Source: CAD feature listing. Evaluate the final solid. Frame: model axes, mm. Face numbers are marked on the shaded views. A direction names the side the tool comes from. Coordinates: 2 decimals unless noted, no trailing zeros. Order: outer loops, then holes, each group sorted by start corner. A loop starts at its lowest first (then second) coordinate and runs counter-clockwise, first axis right, second up. Notation, with made-up numbers: (18, -23) - (53, -23) arc R30 cw to (53, 9) - close; hole circle Ø8 at (19.25, 39.25). An arc over 180 degrees is marked (long way). One line per question, with ' | ' between items. Start each with the question number.
(1) Section B-B (z = 4.5). Count the separate pieces of the cut face and the enclosed holes in it, then the cut area to 3 significant figures.
(2) Section A-A (y = 0). Return the cut outline in (x, z), then the cut area to 3 significant figures.
(3) Contact query for flat-ended pins moving along their axis: P1, Ø2, axis at x = 9, y = 8, coming from the -Z side; P2, Ø5, axis at y = -14.5, z = 2, coming from the -X side; P3, Ø6.5, axis at y = 1, z = -0.5, coming from the +X side. Output: stop coordinate, or through.
(4) Access query for the marked faces 5 and 6. Directions: +Z, -Z, +X, -X, +Y, -Y. A direction counts if a zero-diameter tool reaches every point of the face in a straight line with its end or side. Return the directions, or none.
(5) Draft query along Y for the marked faces 1, 2, 3 and 4. Return one class per face: +Y half, -Y half, draft (parallel to the pull), parting line (faces both ways), or undercut.
(6) Line query: line 1 along Z through (x, y) = (-5.55, 0); line 2 along Y through (x, z) = (7, 5.25); line 3 along Y through (x, z) = (13.5, -1.25). Output: solid intervals per line, ascending.
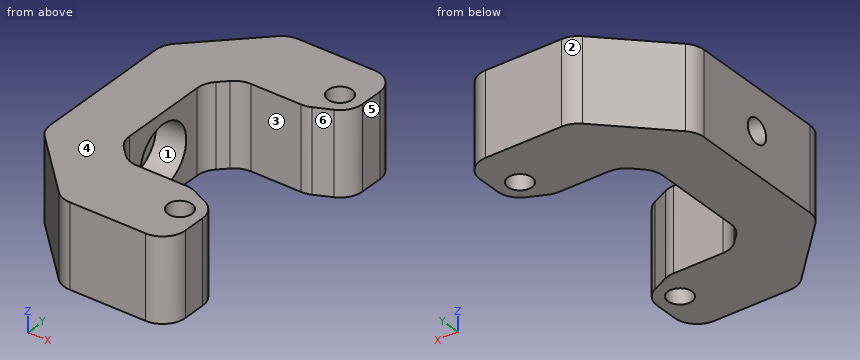
from build123d import *

# Parameters (mm, degrees)
SKETCH_R             = 1.6
PAD_DEPTH            = 5.5
SKETCH001_R          = 1.6
POCKET_DEPTH         = 8.001
POCKET001_DEPTH      = 5.501
POCKET001_DEPTH_BACK = 5.501
SKETCH003_W          = 10
SKETCH003_H          = 45
POCKET002_DEPTH      = 5.501
POCKET002_DEPTH_BACK = 5.501
SKETCH004_R          = 4
POCKET003_DEPTH      = 4
FILLET_R             = 3


with BuildPart() as part:
    # Sketch → Pad (new body, symmetric)
    with BuildSketch(Plane.XY):
        Polygon((1.514719, 20), (18.828427, 20), (18.828427, 10), (6.828427, 10), (2.828427, 10), (0, 7.171573), (0, -7.171573), (2.828427, -10), (6.828427, -10), (18.828427, -10), (18.828427, -20), (1.514719, -20), (-8, -10.485281), (-8, 10.485281), align=None)
        with Locations((12.828427, 14)):
            Circle(SKETCH_R, mode=Mode.SUBTRACT)
        with Locations((12.828427, -14)):
            Circle(SKETCH_R, mode=Mode.SUBTRACT)
    extrude(amount=PAD_DEPTH, both=True)

    # Sketch001 → Pocket (cut, through all)
    with BuildSketch(Plane.YZ):
        Circle(SKETCH001_R)
    extrude(amount=-POCKET_DEPTH, mode=Mode.SUBTRACT)

    # Sketch002 → Pocket001 (cut, two sides)
    with BuildSketch(Plane.XY) as pocket001_sk:
        Polygon((18.828427, 13.487712), (11.349004, 10), (18.828427, 10), align=None)
        Polygon((11.349004, -10), (18.828427, -13.487712), (18.828427, -10), align=None)
    extrude(amount=-POCKET001_DEPTH, mode=Mode.SUBTRACT)
    extrude(pocket001_sk.sketch, amount=POCKET001_DEPTH_BACK, mode=Mode.SUBTRACT)

    # Sketch003 → Pocket002 (cut, two sides)
    with BuildSketch(Plane.XY) as pocket002_sk:
        with Locations((20.828427, 0)):
            Rectangle(SKETCH003_W, SKETCH003_H)
    extrude(amount=-POCKET002_DEPTH, mode=Mode.SUBTRACT)
    extrude(pocket002_sk.sketch, amount=POCKET002_DEPTH_BACK, mode=Mode.SUBTRACT)

    # Sketch004 → Pocket003 (cut)
    with BuildSketch(Plane.YZ):
        Circle(SKETCH004_R)
    extrude(amount=-POCKET003_DEPTH, mode=Mode.SUBTRACT)

    # Fillet
    fillet_edges = [part.edges().sort_by_distance(p)[0] for p in [
        (15.828427, -20, 0),
        (15.828427, -12.088789, 0),
        (11.349004, -10, 0),
        (2.828427, -10, 0),
        (0, -7.171573, 0),
        (0, 7.171573, 0),
        (2.828427, 10, 0),
        (11.349004, 10, 0),
        (15.828427, 12.088789, 0),
        (15.828427, 20, 0),
        (1.514719, 20, 0),
        (-8, 10.485281, 0),
        (-8, -10.485281, 0),
        (1.514719, -20, 0),
    ]]
    fillet(fillet_edges, radius=FILLET_R)


solid = part.part
Response values:
1) separate pieces: 1 | enclosed holes: 2 | area: 523 mm²
2) outline: (-8, -5.5) - (0, -5.5) - (0, -4) - (-4, -4) - (-4, -1.6) - (-8, -1.6) - close; (-8, 1.6) - (-4, 1.6) - (-4, 4) - (0, 4) - (0, 5.5) - (-8, 5.5) - close | area: 43.2 mm²
3) P1: passes through | P2: stops at x = -6.49 | P3: stops at x = 0
4) face 5: +Z, -Z, +X, +Y, -Y | face 6: +Z, -Z, +X
5) face 1: undercut | face 2: +Y half | face 3: undercut | face 4: draft
6) line 1: z = -5.5 to -1.6, 1.6 to 5.5 | line 2: y = -20 to -10, 10 to 20 | line 3: y = -19.92 to -15.45, -12.55 to -11, 11 to 12.55, 15.45 to 19.92
